Model file for the job. Use its own axes, mm. A direction names the side the tool comes from. Round coordinates to 2 decimals unless told otherwise and drop trailing zeros. Order: outer loops, then holes, each group sorted by start corner. A loop starts at its lowest first (then second) coordinate and runs counter-clockwise, first axis right, second up. Notation, with made-up numbers: (-11, 20) - (-5, 20) arc R7 ccw to (-5, 25) - close; hole circle Ø9 at (84.5, 49.5). An arc over 180 degrees is marked (long way). Put each result on its own line as item: value. Start each with the question number.
Item 1: Which spindle directions (+Z, -Z, +X, -X, +Y, -Y) get a long thin tool onto all of the face, cutting with end or side? Do faces 4 (the face through (-15.26, -3.49, 3.25)), 5 (the face through (-21, 9, 3.5)). Say none if no direction does.
Item 2: Pin check, flat tips, straight feed: pin 1 Ø1.5 at (y, z) = (45.5, 1.5) entering from +X; pin 2 Ø1.5 at (y, z) = (-39.5, 1.5) entering from -X; pin 3 Ø2 at (x, z) = (52.5, 1.5) entering from +Y. Stop position of each tip, or through.
Item 3: Probe probe 1 along Y at (x, z) = (0.5, 0.95); probe 2 along Z at (x, y) = (-7.5, 0.5); probe 3 along X at (y, z) = (23.5, 1.55). List the from-to ranges inside material, lowest first.
Item 4: Mould opens along Y. For faces 1 (the face through (63, 19.8, 0.7)), 2 (the face through (-16.845, -25.311, 3.254)), 3 (the face through (13, 1, 3.5)) say: pulls with the +Y half, pulls with the -Y half, needs draft (parallel to the pull), parting line crosses it, or undercut.
Item 5: Saw through at A-A on z = 0.9. List the corners of the cut face in (x, y).
```python
from build123d import *

# Parameters (mm, degrees)
F0_R     = 66.04
F1_DEPTH = 3.5
F3_DEPTH = 0.5
F4_R     = 2


with BuildPart() as f1:
    # F0 (on Top) → F1 (new body)
    with BuildSketch(Plane.XY):
        Circle(F0_R)
    extrude(amount=F1_DEPTH)

    # F2 (on face) → F3 (cut)
    with BuildSketch(Plane.XY.offset(3.5)):
        with BuildLine():
            Line((36.7589145899, 37.629019469), (7.088160608, 29.8062227666))
            add(Edge.make_bspline(
                [(-27.9188621789, -24.7298497707), (-28.6586928586, -24.2103901464), (-30.4148624686, -22.977325297), (-34.7839086401, -19.2292372163), (-36.7492639554, -15.8301967621), (-38.5813905625, -12.392258781), (-39.75259532, -7.49957565), (-39.8114737138, -2.8913390892), (-39.4153051917, 1.3872774793), (-37.155174617, 6.8463574778), (-34.2487020488, 11.5543521179), (-30.1449211522, 16.1966267345), (-24.8865606472, 20.5465305085), (-18.820652323, 23.9222079865), (-13.5893033373, 26.3447324713), (-6.2676210393, 28.8086948244), (-0.9973036761, 29.4594702935), (2.8494568659, 29.9332388479), (5.6501959782, 29.8493125043), (7.088160608, 29.8062227666)],
                knots=[0, 0, 0, 0, 0.0451249272, 0.1071150846, 0.1588573068, 0.2095718144, 0.267664136, 0.3232882023, 0.3768767861, 0.4394121671, 0.5007893365, 0.5650325207, 0.6332195526, 0.7010771123, 0.7641179487, 0.8361406793, 0.8960766014, 0.946643309, 1, 1, 1, 1], degree=3))
            Line((-27.9188621789, -24.7298497707), (-38.6472716928, -37.1904484928))
            add(Edge.make_bspline(
                [(8.680658415, -1.9040451152), (-7.0953182876, -13.6661795744), (-22.8712949902, -25.4283140336), (-38.6472716928, -37.1904484928)],
                knots=[0, 0, 0, 0, 59.0344241236, 59.0344241236, 59.0344241236, 59.0344241236], degree=3))
            Line((8.680658415, -1.9040451152), (-3.7240635138, -4.4464543462))
            Line((-3.7240635138, -4.4464543462), (24.2703761905, 18.8822448254))
            Line((24.2703761905, 18.8822448254), (11.5583296865, 17.3176843673))
            Line((11.5583296865, 17.3176843673), (36.7589145899, 37.629019469))
        make_face()
        with BuildLine():
            add(Edge.make_bspline(
                [(3.7381993607, 27.1198898554), (2.971135623, 27.1618474152), (1.2947530215, 27.2535437369), (-1.9863245634, 26.752964039), (-5.5830102518, 26.3936384961), (-8.1626603235, 25.6625858195), (-11.8819068257, 24.5992540716), (-15.194299707, 23.2915717189), (-18.3387248736, 21.7834257182), (-22.657889275, 19.4908286459), (-25.3334584396, 17.405984417), (-28.4560760539, 14.5877478565), (-31.1520888031, 11.8106881463), (-33.1981293641, 8.6361921113), (-34.8489244867, 5.4336172817), (-35.6717957614, 1.8976307489), (-36.1212606559, -0.7356813567), (-36.1055273874, -4.9327401117), (-35.284250801, -7.7228924909), (-33.7690554357, -11.151243353), (-31.7825018341, -13.6634363898), (-29.4483207392, -15.9985267381), (-27.0119624763, -17.7648035422), (-25.4106160526, -18.7590652994), (-24.3846229373, -19.3770721413), (-23.8800570369, -19.6809973568)],
                knots=[0, 0, 0, 0, 0.0370080786, 0.0808794576, 0.1262134195, 0.1655943936, 0.2123656254, 0.2575173754, 0.3025728065, 0.3550686508, 0.3996737986, 0.4482930207, 0.4956445603, 0.5418786203, 0.587545708, 0.6324346113, 0.6721602243, 0.720331977, 0.7617849857, 0.8074577834, 0.8504872685, 0.8941300827, 0.9355240772, 0.9682918418, 1, 1, 1, 1], degree=3))
            Line((3.7381993607, 27.1198898554), (-15.5056634386, 5.2878007289))
            Line((-15.5056634386, 5.2878007289), (-4.4998652302, 6.9099701941))
            Line((-4.4998652302, 6.9099701941), (-26.3297446072, -14.188955538))
            Line((-26.3297446072, -14.188955538), (-17.6175478846, -12.9048451781))
            Line((-17.6175478846, -12.9048451781), (-23.8800570369, -19.6809973568))
        make_face(mode=Mode.SUBTRACT)
        with BuildLine():
            add(Edge.make_bspline(
                [(23.0140855235, 22.1223023413), (23.6337480093, 21.7049911427), (25.0817865454, 20.7298107649), (28.3144677633, 17.8145217038), (30.5631850073, 14.3623327366), (31.9299956157, 11.4542653938), (32.4038757117, 8.878719599), (32.7918336503, 5.3554549599), (32.1630546429, 0.8710537681), (30.7342580485, -2.9112662617), (28.7888202269, -6.4806965762), (25.7872064292, -9.7882796528), (23.0901008337, -12.5984417239), (20.3259832239, -14.8008398541), (16.8563718909, -16.7655352132), (12.083012982, -19.4120821964), (6.6545909805, -21.2312151302), (2.6297224287, -22.1259203281), (-2.7686651604, -23.1002452156), (-11.2544630445, -23.2923264004), (-12.8249440359, -22.861325742), (-13.338916935, -22.7202717215)],
                knots=[0, 0, 0, 0, 0.0405040979, 0.0946507106, 0.1480773568, 0.1940198869, 0.2355227836, 0.2842322816, 0.3395597185, 0.3918333536, 0.4440264689, 0.4989766927, 0.5503408725, 0.5986057845, 0.650215388, 0.7114530865, 0.7735610236, 0.8254499534, 0.8879083382, 0.9633156487, 1, 1, 1, 1], degree=3))
            Line((-13.338916935, -22.7202717215), (-20.4509142786, -27.9752481729))
            add(Edge.make_bspline(
                [(-20.4509142786, -27.9752481729), (-18.8172337543, -28.4739563845), (-15.4699105031, -29.4957826029), (-9.8113094816, -30.5934467075), (-3.4476646051, -30.5276095836), (3.8323637699, -29.7792821906), (10.9948418748, -28.1270192234), (18.1616670883, -25.4269070755), (24.9613540992, -21.2618874253), (29.7707603508, -17.7083655535), (34.6400151481, -12.6535211177), (38.1350855825, -7.1300397484), (39.906954757, -2.6337329233), (40.7854535947, 1.4807883485), (40.3205082437, 6.8263907972), (39.2885733015, 12.3641756391), (35.9753768895, 17.0850121131), (32.6981331654, 20.6047877337), (28.1143591936, 23.9871411799), (26.8914743312, 24.6504593747), (26.4487545937, 24.8905997723)],
                knots=[0, 0, 0, 0, 0.0528863325, 0.1083612418, 0.1669825339, 0.2298350138, 0.2928105097, 0.3573840476, 0.4226321743, 0.4795914908, 0.5409064156, 0.6005080495, 0.6510696648, 0.6981285603, 0.7516560544, 0.8069216428, 0.8617149771, 0.914131578, 0.9689131443, 1, 1, 1, 1], degree=3))
            Line((26.4487545937, 24.8905997723), (23.0140855235, 22.1223023413))
        make_face()
    extrude(amount=-F3_DEPTH, mode=Mode.SUBTRACT)

    # F4
    f4_edges = [f1.edges().sort_by_distance(p)[0] for p in [
        (-66.04, 0, 3.5),
    ]]
    fillet(f4_edges, radius=F4_R)


solid = f1.part
```
Results found:
1. face 4: +Z
1. face 5: +Z, +X, -X, +Y, -Y
2. pin 1: stops at x = 48.57
2. pin 2: stops at x = -53.48
2. pin 3: stops at y = 41.34
3. probe 1: y = -66.04 to 66.04
3. probe 2: z = 0 to 3
3. probe 3: x = -61.72 to 61.72
4. face 1: parting line crosses it
4. face 2: undercut
4. face 3: needs draft
5. outline: circle Ø132.08 at (0, 0)
